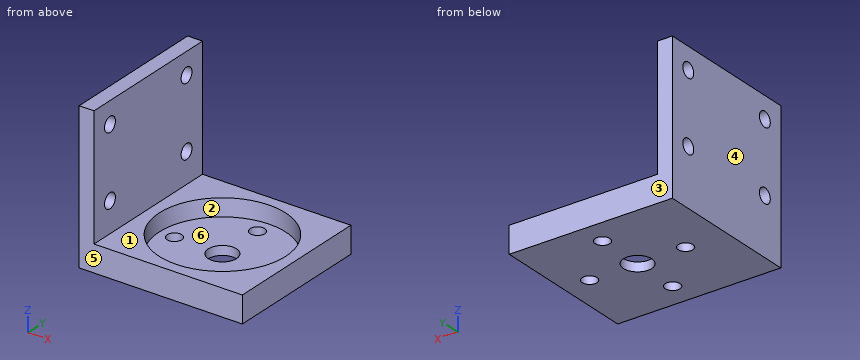
```python
from build123d import *

# Parameters (mm, degrees)
SKETCH1_W            = 34
SKETCH1_H            = 34
BOSS_EXTRUDE1_DEPTH  = 6.08
SKETCH2_W            = 34
SKETCH2_H            = 34
BOSS_EXTRUDE2_DEPTH  = 3.4
HOLE1_D              = 3.4
SKETCH5_R            = 14.5
CUT_EXTRUDE1_DEPTH   = 4
M3_CLEARANCE_HOLE1_D = 3.4
HOLE2_D              = 6.5


with BuildPart() as part:
    # Sketch1 → Boss-Extrude1 (new body)
    with BuildSketch(Plane(origin=(0, 0, 0), x_dir=(0, 1, 0), z_dir=(0, 0, 1))):
        with Locations((17, 17)):
            Rectangle(SKETCH1_W, SKETCH1_H)
    extrude(amount=BOSS_EXTRUDE1_DEPTH)

    # Sketch2 → Boss-Extrude2 (add)
    with BuildSketch(Plane(origin=(-34, 0, 0), x_dir=(0, -1, 0), z_dir=(-1, 0, 0))):
        with Locations((-17, 17)):
            Rectangle(SKETCH2_W, SKETCH2_H)
    extrude(amount=BOSS_EXTRUDE2_DEPTH)

    # Hole1 (through all)
    with Locations(Plane.YZ.offset(-34)):
        with Locations((5, 29), (29, 29), (5, 13), (29, 13)):
            Hole(HOLE1_D / 2)

    # Sketch5 → Cut-Extrude1 (cut)
    with BuildSketch(Plane.XY.offset(6.08)):
        with Locations((-17, 17)):
            Circle(SKETCH5_R)
    extrude(amount=-CUT_EXTRUDE1_DEPTH, mode=Mode.SUBTRACT)

    # M3 Clearance Hole1 (through all)
    with Locations(Plane(origin=(0, 0, 2.08), x_dir=(0, -1, 0), z_dir=(0, 0, 1))):
        with Locations((-17, -6), (-6, -17), (-17, -28), (-28, -17)):
            Hole(M3_CLEARANCE_HOLE1_D / 2)

    # Hole2 (through all)
    with Locations(Plane(origin=(0, 0, 2.08), x_dir=(0, -1, 0), z_dir=(0, 0, 1))):
        with Locations((-17, -17)):
            Hole(HOLE2_D / 2)


solid = part.part
```
Check sheet for the modelled part. Datum: model origin and axes. Units: mm. Face numbers are marked on the shaded views. A direction names the side the tool comes from. Give positions to 0.01 mm unless a question says otherwise; leave off trailing zeros. Loops run counter-clockwise (first coordinate to the right, second up) from the corner with the lowest first, then second, coordinate; pieces in that order, holes last. Notation, with made-up numbers: M 63.5,22.5 L 100.5,22.5 A27 ccw 100.5,49.5 Z; hole C -2.5,40 d7. An arc over 180 degrees is marked long. Answer as CSV lines item,"result".
Item 1: Scan lines: L1, parallel to X at y = 17, z = 1.1; L2, parallel to Z at x = -35, y = 29; L3, parallel to X at y = 23, z = 29. Record each from-to range of solid material in increasing order.
Reply:
L1,"-37.4 to -29.7, -26.3 to -20.25, -13.75 to -7.7, -4.3 to 0"
L2,"0 to 11.3, 14.7 to 27.3, 30.7 to 34"
L3,"-37.4 to -34"
Item 2: Sectioned sample at A-A, the plane y = 17. Enter the section's corners in (x, z).
Reply:
outline,"M -37.4,0 L -29.7,0 L -29.7,2.08 L -31.5,2.08 L -31.5,6.08 L -34,6.08 L -34,34 L -37.4,34 Z; M -26.3,0 L -20.25,0 L -20.25,2.08 L -26.3,2.08 Z; M -13.75,0 L -7.7,0 L -7.7,2.08 L -13.75,2.08 Z; M -4.3,0 L 0,0 L 0,6.08 L -2.5,6.08 L -2.5,2.08 L -4.3,2.08 Z"
Item 3: Sectioned sample at D-D, the plane x = -34.5. Enter the section's corners in (y, z), then the cut area to 3 significant figures.
Reply:
outline,"M 0,0 L 34,0 L 34,34 L 0,34 Z; hole C 5,13 d3.4; hole C 5,29 d3.4; hole C 29,13 d3.4; hole C 29,29 d3.4"
area,"1,120 mm^2"
Item 4: Sectioned sample at B-B, the plane x = -17. Enter the section's corners in (y, z).
Reply:
outline,"M 0,0 L 4.3,0 L 4.3,2.08 L 2.5,2.08 L 2.5,6.08 L 0,6.08 Z; M 7.7,0 L 13.75,0 L 13.75,2.08 L 7.7,2.08 Z; M 20.25,0 L 26.3,0 L 26.3,2.08 L 20.25,2.08 Z; M 29.7,0 L 34,0 L 34,6.08 L 31.5,6.08 L 31.5,2.08 L 29.7,2.08 Z"
Item 5: Depth check by flat-ended pin: pin 1 Ø12 at (y, z) = (12.5, 19.5) entering from +X; pin 2 Ø17 at (x, y) = (-9, 14) entering from +Z; pin 3 Ø4 at (x, y) = (-17, 28) entering from +Z. Enter the tip coordinate at first touch or a pass-through.
Reply:
pin 1,"x = -34"
pin 2,"z = 6.08"
pin 3,"z = 2.08"
Item 6: Set-up check for the marked faces 1, 2 and 3: record each of +Z, -Z, +X, -X, +Y, -Y from which the full face is reachable in a straight line by a thin tool's end or side.
Reply:
face 1,"+Z, +X, +Y, -Y"
face 2,"+Z"
face 3,"+Z, -Z, +X, -X, +Y"
Item 7: Draft check along X on the marked faces 4, 5 and 6. Enter one of: pulls with the +X half, pulls with the -X half, needs draft (parallel to the pull), parting line crosses it, or undercut.
Reply:
face 4,"pulls with the -X half"
face 5,"needs draft"
face 6,"undercut"
Item 8: Sectioned sample at C-C, the plane z = 13. Enter the section's corners in (x, y), then the cut area to 3 significant figures.
Reply:
outline,"M -37.4,0 L -34,0 L -34,3.3 L -37.4,3.3 Z; M -37.4,6.7 L -34,6.7 L -34,27.3 L -37.4,27.3 Z; M -37.4,30.7 L -34,30.7 L -34,34 L -37.4,34 Z"
area,"92.5 mm^2"
